For this review, take the finished solid that the model builds, in its own axes (mm). A direction names the side the tool comes from. Round coordinates to 2 decimals unless told otherwise and drop trailing zeros. Loops run counter-clockwise (first coordinate to the right, second up) from the corner with the lowest first, then second, coordinate; pieces in that order, holes last. Notation, with made-up numbers: (-21, -18.75) -> (25, -18.75) arc R24 ccw to (25, 18.25) -> close; hole circle Ø10 at (76.25, 76.5). An arc over 180 degrees is marked (long way). One line per question, with ' | ' between items. Start each with the question number.
1. Consider section A-A (z = 3). Write out the cut boundary in (x, y).
2. Draft analysis for pull direction Y (two halves, no side actions). For faces 3 (the face through (0, 0, -4)), 4 (the face through (-0.07, -1.5, -0.67)), 5 (the face through (1, 0, 3)), 6 (the face through (0.51, 0.86, 3.41)), state which applies: pulls with the +Y half, pulls with the -Y half, needs draft (parallel to the pull), parting line crosses it, or undercut.
3. Wall thickness on line 1 along Y through (x, z) = (-0.05, -0.5); line 2 along Z through (x, y) = (-0.4, 0.6); line 3 along Z through (x, y) = (1.1, 1.4): over which ranges is each line inside the solid? List them lowest first.
4. For faces 1 (the face through (-1, 0, 3)), 2 (the face through (1, -1, 4)), list the 3-axis set-ups (+Z, -Z, +X, -X, +Y, -Y) from which the entire face can be reached by the end or side of a thin tool; tool diameter is ignored.
5. For pin 1 Ø1 at (x, y) = (1.5, -1) entering from -Z; pin 2 Ø1.6 at (x, y) = (0.5, 0.5) entering from +Z; pin 3 Ø1 at (y, z) = (1.5, 2) entering from +X, all flat-tipped, find the tip position at first contact; note any pin that passes through.
6. Consider section B-B (y = 0). Write out the cut boundary in (x, z).
7. Consider section C-C (z = -0.5). Write out the cut boundary in (x, y).
```python
from build123d import *

# Parameters (mm, degrees)
SKETCH3_W          = 8
SKETCH3_H          = 1.5
CHAMFER1_SIZE      = 0.45
CUT_EXTRUDE1_DEPTH = 1.19


with BuildPart() as part:
    # Sketch3 → Revolve1 (revolve)
    with BuildSketch(Plane(origin=(0, 0, 0), x_dir=(0, 0, -1), z_dir=(1, 0, 0))):
        with Locations((0, 0.75)):
            Rectangle(SKETCH3_W, SKETCH3_H)
    revolve(axis=Axis((0, 0, -4), (0, 0, 1)))

    # Chamfer1
    chamfer1_edges = [part.edges().sort_by_distance(p)[0] for p in [
        (0, -1.5, -4),
    ]]
    chamfer(chamfer1_edges, length=CHAMFER1_SIZE)

    # Sketch6 → Revolve2 (revolve)
    with BuildSketch(Plane(origin=(0, 0, 0), x_dir=(0, 0, -1), z_dir=(1, 0, 0))):
        Polygon((-4, 3), (-3.8, 3), (-2.3, 1.5), (-2.3, 0), (-4, 0), align=None)
    revolve(axis=Axis((0, 0, -4), (0, 0, 1)))

    # Sketch8 → Cut-Extrude1 (cut)
    with BuildSketch(Plane.XY.offset(4)):
        Polygon((0, 1.154700538), (-1, 0.577350269), (-1, -0.577350269), (0, -1.154700538), (1, -0.577350269), (1, 0.577350269), align=None)
    extrude(amount=-CUT_EXTRUDE1_DEPTH, mode=Mode.SUBTRACT)

    # Cut-Extrude2 cone 1 section (through the dimple's axis) → Cut-Extrude2 (revolve, cut)
    with BuildSketch(Plane(origin=(0, 0, 4), x_dir=(0, -1, 0), z_dir=(1, 0, 0))):
        Polygon((0, 0), (1.154700538, 0), (0, 1.154700538), align=None)
    revolve(axis=Axis((0, 0, 4), (0, 0, -1)), mode=Mode.SUBTRACT)


solid = part.part
```
Answer block:
1) outline: circle Ø4.4 at (0, 0); hole (-1, -0.58) -> (0, -1.15) -> (1, -0.58) -> (1, 0.58) -> (0, 1.15) -> (-1, 0.58) -> close
2) face 3: needs draft | face 4: parting line crosses it | face 5: undercut | face 6: undercut
3) line 1: y = -1.5 to 1.5 | line 2: z = -4 to 2.81 | line 3: z = 2.58 to 4
4) face 1: +Z | face 2: +Z, +X, -X, +Y, -Y
5) pin 1: stops at z = -3.75 | pin 2: stops at z = 4 | pin 3: stops at x = 1.12
6) outline: (-3, 3.8) -> (-1.5, 2.3) -> (-1.5, -3.55) -> (-1.05, -4) -> (1.05, -4) -> (1.5, -3.55) -> (1.5, 2.3) -> (3, 3.8) -> (3, 4) -> (1.15, 4) -> (1, 3.85) -> (1, 2.81) -> (-1, 2.81) -> (-1, 3.85) -> (-1.15, 4) -> (-3, 4) -> close
7) outline: circle Ø3 at (0, 0)
